```python
from build123d import *

# Parameters (mm, degrees)
SKETCH3_W          = 4.030508652
SKETCH3_H          = 4.030508652
SKETCH3_W_2        = 2.295648056
SKETCH3_H_2        = 0.7
CUT_EXTRUDE1_DEPTH = 8
CHAMFER1_SIZE      = 1
FILLET1_R          = 0.5


with BuildPart() as part:
    # Sketch2 → Revolve1 (revolve)
    with BuildSketch(Plane(origin=(0, 0, 0), x_dir=(0, 0, -1), z_dir=(1, 0, 0))):
        Polygon((0, 1), (12, 1), (12, 0), (24, 0), (24, 1.2), (16, 1.2), (16, 2.85), (3, 2.85), (3, 3.605), (0, 3.605), align=None)
    revolve(axis=Axis((0, 0, 0), (0, 0, -1)))

    # Sketch3 → Cut-Extrude1 (cut)
    with BuildSketch(Plane(origin=(0, 0, -24), x_dir=(-1, 0, 0), z_dir=(0, 0, -1))):
        Rectangle(SKETCH3_W, SKETCH3_H)
        Rectangle(SKETCH3_W_2, SKETCH3_H_2, mode=Mode.SUBTRACT)
    extrude(amount=-CUT_EXTRUDE1_DEPTH, mode=Mode.SUBTRACT)

    # Chamfer1
    chamfer1_edges = [part.edges().sort_by_distance(p)[0] for p in [
        (0, -1, 0),
    ]]
    chamfer(chamfer1_edges, length=CHAMFER1_SIZE)

    # Fillet1
    fillet1_edges = [part.edges().sort_by_distance(p)[0] for p in [
        (0, -2, 0),
        (0, -3.605, 0),
        (0, -2.85, -16),
    ]]
    fillet(fillet1_edges, radius=FILLET1_R)


solid = part.part
```
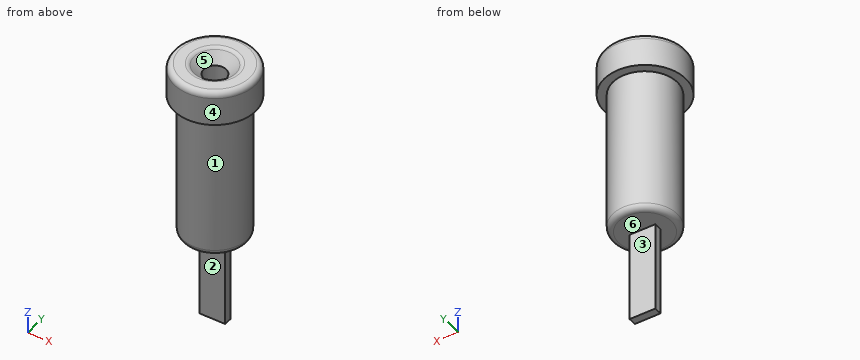
Input: part model. Units: mm. Frame: model coordinates. Face numbers are marked on the shaded views. A direction names the side the tool comes from. Give positions to 0.01 mm unless a question says otherwise; leave off trailing zeros. Order: outer loops, then holes, each group sorted by start corner. A loop starts at its lowest first (then second) coordinate and runs counter-clockwise, first axis right, second up. Notation, with made-up numbers: (77, 88.5) - (130, 88.5) arc R23 ccw to (130, 116.5) - close; hole circle Ø8 at (74, -21). An arc over 180 degrees is marked (long way). Use a Markdown table: item, result.
(1) Section query B-B (x = 0). Output: boundary loops of the cut face in (y, z) (3 decimals), then the cut area to 3 significant figures.
Computed values:
| item | result |
|---|---|
| outline | (-3.605, -3) - (-2.85, -3) - (-2.85, -15.5) arc R0.5 ccw to (-2.35, -16) - (-0.35, -16) - (-0.35, -24) - (0.35, -24) - (0.35, -16) - (2.35, -16) arc R0.5 ccw to (2.85, -15.5) - (2.85, -3) - (3.605, -3) - (3.605, -0.5) arc R0.5 ccw to (3.105, 0) - (2.207, 0) arc R0.5 ccw to (1.854, -0.146) - (1, -1) - (1, -12) - (-1, -12) - (-1, -1) - (-1.854, -0.146) arc R0.5 ccw to (-2.207, 0) - (-3.105, 0) arc R0.5 ccw to (-3.605, -0.5) - close |
| area | 76.1 mm2 |
(2) Section query A-A (y = 0). Output: boundary loops of the cut face in (x, z) (3 decimals).
Computed values:
| item | result |
|---|---|
| outline | (-3.605, -3) - (-2.85, -3) - (-2.85, -15.5) arc R0.5 ccw to (-2.35, -16) - (-1.148, -16) - (-1.148, -24) - (1.148, -24) - (1.148, -16) - (2.35, -16) arc R0.5 ccw to (2.85, -15.5) - (2.85, -3) - (3.605, -3) - (3.605, -0.5) arc R0.5 ccw to (3.105, 0) - (2.207, 0) arc R0.5 ccw to (1.854, -0.146) - (1, -1) - (1, -12) - (-1, -12) - (-1, -1) - (-1.854, -0.146) arc R0.5 ccw to (-2.207, 0) - (-3.105, 0) arc R0.5 ccw to (-3.605, -0.5) - close |
(3) Section query C-C (z = -17.5). Output: boundary loops of the cut face in (x, y).
Computed values:
| item | result |
|---|---|
| outline | (-1.15, -0.35) - (1.15, -0.35) - (1.15, 0.35) - (-1.15, 0.35) - close |
(4) Draft query along X for the marked faces 4, 5 and 6. Return one class per face: released by +X, released by -X, zero draft, split by the parting line, or undercut.
Computed values:
| item | result |
|---|---|
| face 4 | split by the parting line |
| face 5 | undercut |
| face 6 | zero draft |
(5) Line query: line 1 (X direction, y = 0, z = -11.5); line 2 (Y direction, x = 0, z = -16.5); line 3 (Y direction, x = -0.75, z = -6). Output: solid intervals per line, ascending. Write a range as from..to.
Computed values:
| item | result |
|---|---|
| line 1 | x = -2.85..-1, 1..2.85 |
| line 2 | y = -0.35..0.35 |
| line 3 | y = -2.75..-0.66, 0.66..2.75 |
(6) Access query for the marked faces 1, 2 and 3. Directions: +Z, -Z, +X, -X, +Y, -Y. A direction counts if a zero-diameter tool reaches every point of the face in a straight line with its end or side. Return the directions, or none.
Computed values:
| item | result |
|---|---|
| face 1 | -Z |
| face 2 | -Z, +X, -X, -Y |
| face 3 | -Z, +X, -X, +Y |
(7) Pin query (flat end, axial travel): pin 1 (4 mm diameter, centred on y = 0.5, z = -8, fed in from -X); pin 2 (1.1 mm diameter, centred on x = 0.5, z = -20, fed in from -Y); pin 3 (4 mm diameter, centred on y = -0.5, z = -6, fed in from +X). Return the tip coordinate at first contact, or that it passes through.
Computed values:
| item | result |
|---|---|
| pin 1 | stops at x = -2.85 |
| pin 2 | stops at y = -0.35 |
| pin 3 | stops at x = 2.85 |
